from build123d import *

# Parameters (mm, degrees)
F4_DEPTH = 3.176
F5_SIZE  = 1.016


# Not quite as in the source:
# - a fillet or chamfer that OpenCascade refuses, or shapes differently, is made with other operations: its cross-section is extruded or revolved along the edge and cut away or added


with BuildPart() as f1:
    # F0 (on Front) → F1 (revolve)
    with BuildSketch(Plane.XZ):
        with BuildLine():
            Line((3.175, 0), (5.715, 0))
            ThreePointArc((5.715, 0), (3.2688625698, 2.3279526256), (0, 3.175))
            Line((0, 3.175), (0, -12.7))
            Line((0, -12.7), (3.175, -12.7))
            Line((3.175, -12.7), (3.175, 0))
        make_face()
    revolve(axis=Axis((0, 0, -4.7625), (0, 0, 1)))

    # F2: chamfer of 0.762 on 1 edges, made by hand

    # F2_s1 → F2_t2 (revolve, cut)
    with BuildSketch(Plane.XZ):
        with BuildLine():
            Line((4.8809391349, -0.0275238998), (5.2355867217, 0.7179265843))
            Line((5.2355867217, 0.7179265843), (5.2474112325, 0.727541081))
            ThreePointArc((5.2474112325, 0.727541081), (5.4877257432, 0.3678527374), (5.7279396226, 0.0080513208))
            Line((5.7279396226, 0.0080513208), (5.715, -0.01524))
            ThreePointArc((5.715, -0.01524), (5.2979695675, -0.01524), (4.8809391349, -0.0427638998))
            Line((4.8809391349, -0.0427638998), (4.8809391349, -0.0275238998))
        make_face()
    revolve(axis=Axis((0, 0, 0), (0, 0, 1)), mode=Mode.SUBTRACT)

    # F3 (on Top) → F4 (cut, through all)
    with BuildSketch(Plane.XY):
        Polygon((0.635, 2.54), (-0.635, 2.54), (-0.635, 0.635), (-2.54, 0.635), (-2.54, -0.635), (-0.635, -0.635), (-0.635, -2.54), (0.635, -2.54), (0.635, -0.635), (2.54, -0.635), (2.54, 0.635), (0.635, 0.635), align=None)
    extrude(amount=F4_DEPTH, mode=Mode.SUBTRACT)

    # F5
    f5_edges = [f1.edges().sort_by_distance(p)[0] for p in [
        (-3.175, 0, -12.7),
    ]]
    chamfer(f5_edges, length=F5_SIZE)


solid = f1.part
Model file for the job. Use its own axes, mm. A direction names the side the tool comes from. Give positions to 0.01 mm unless a question says otherwise; leave off trailing zeros. Order: outer loops, then holes, each group sorted by start corner. A loop starts at its lowest first (then second) coordinate and runs counter-clockwise, first axis right, second up. Notation, with made-up numbers: (3, -38.5) - (31, -38.5) arc R19 cw to (31, -30.5) - close; hole circle Ø7 at (-38, -27). An arc over 180 degrees is marked (long way). One line per item, written item: value.
Item 1: Two-plate mould, pull along Y, no slides. Class faces 1 (the flat face through (-1, -3.2, 0)), 2 (the flat face through (-0.635, -2, 2)), 3 (the cylindrical face through (-0.69, -3.1, -5.76)): released by +Y, released by -Y, zero draft, split by the parting line, or undercut.
Response values:
face 1: zero draft
face 2: undercut
face 3: split by the parting line
Item 2: Slice it at A-A (x = 0). List the corners of the cut face in (y, z) (1 decimal).
Response values:
outline: (-5.2, 0.7) - (-4.9, 0) - (-3.2, 0) - (-3.2, -11.7) - (-2.2, -12.7) - (2.2, -12.7) - (3.2, -11.7) - (3.2, 0) - (4.9, 0) - (5.2, 0.7) arc R6.7 ccw to (2.5, 2.7) - (2.5, 0) - (-2.5, 0) - (-2.5, 2.7) arc R6.7 ccw to start
Item 3: Wall check: line 1 (Y direction, x = 0.25, z = 1.5); line 2 (Z direction, x = 0.5, y = -0.5); line 3 (Y direction, x = -2.75, z = 1.5). Give the ranges that are in metal, low to high.
Response values:
line 1: -4.44 to -2.54, 2.54 to 4.44
line 2: -12.7 to 0
line 3: -3.49 to 3.49
Item 4: Tool access for faces 4 (the flat face through (0, 0, -12.7)), 5 (the flat face through (2, -0.635, 2)): list every direction of +Z, -Z, +X, -X, +Y, -Y with a clear straight run to the whole face (end or side of a thin tool).
Response values:
face 4: -Z, +X, -X, +Y, -Y
face 5: +Z
Item 5: Slice it at C-C (z = -0.75). List the corners of the cut face in (x, y) (3 decimals), then the cut area to 3 significant figures.
Response values:
outline: circle Ø6.35 at (0, 0)
area: 31.7 mm2
Item 6: Pin check, flat tips, straight feed: pin 1 Ø2 at (y, z) = (-1.5, 1) entering from -X; pin 2 Ø0.6 at (x, z) = (-2, 1.5) entering from +Y; pin 3 Ø0.6 at (x, z) = (1.5, 2.5) entering from -Y; pin 4 Ø1.4 at (x, z) = (0, 1) entering from +Y. Stop position of each tip, or through.
Response values:
pin 1: x = -5.19
pin 2: y = 4.35
pin 3: y = -3.17
pin 4: y = 5.22
